Source: CAD feature listing. Evaluate the final solid. Frame: model axes, mm. A direction names the side the tool comes from. Give positions to 0.01 mm unless a question says otherwise; leave off trailing zeros. Order: outer loops, then holes, each group sorted by start corner. A loop starts at its lowest first (then second) coordinate and runs counter-clockwise, first axis right, second up.
from build123d import *

# Parameters (mm, degrees)
PAD_DEPTH       = 4
POCKET_DEPTH    = 1
POCKET001_DEPTH = 3.001


with BuildPart() as part:
    # Sketch → Pad (new body)
    with BuildSketch(Plane.XY):
        with BuildLine():
            Line((0, 0), (50, 0))
            ThreePointArc((50, 0), (62.5, 12.5), (50, 25))
            Line((50, 25), (0, 25))
            ThreePointArc((0, 25), (-12.5, 12.5), (0, 0))
        make_face()
    extrude(amount=PAD_DEPTH)

    # Sketch001 (on Face6 of Pad) → Pocket (cut)
    with BuildSketch(Plane.XY.offset(4)):
        with BuildLine():
            Line((0, 2), (50, 2))
            ThreePointArc((50, 2), (60.5, 12.5), (50, 23))
            Line((50, 23), (0, 23))
            ThreePointArc((0, 23), (-10.5, 12.5), (0, 2))
        make_face()
    extrude(amount=-POCKET_DEPTH, mode=Mode.SUBTRACT)

    # Sketch002 (on Face11 of Pocket) → Pocket001 (cut, through all)
    with BuildSketch(Plane.XY.offset(3)):
        with BuildLine():
            ThreePointArc((-2, 17.5), (-4.5, 20), (-7, 17.5))
            Line((-7, 17.5), (-7, 7.5))
            ThreePointArc((-7, 7.5), (-4.5, 5), (-2, 7.5))
            Line((-2, 7.5), (-2, 17.5))
        make_face()
    extrude(amount=-POCKET001_DEPTH, mode=Mode.SUBTRACT)


solid = part.part
1) Section query A-A on y = 12.5. Output: boundary loops of the cut face in (x, z), and give its area (3 significant figures).
Checks:
outline: (-12.5, 0) - (-7, 0) - (-7, 3) - (-10.5, 3) - (-10.5, 4) - (-12.5, 4) - close; (-2, 0) - (62.5, 0) - (62.5, 4) - (60.5, 4) - (60.5, 3) - (-2, 3) - close
area: 214 mm2
2) Section query C-C on x = -4.5. Output: boundary loops of the cut face in (y, z).
Checks:
outline: (0.84, 0) - (5, 0) - (5, 3) - (3.01, 3) - (3.01, 4) - (0.84, 4) - close; (20, 0) - (24.16, 0) - (24.16, 4) - (21.99, 4) - (21.99, 3) - (20, 3) - close
3) Reachability of faces 1 (the face through (25, 0, 2)), 2 (the face through (25, 13, 3)), 3 (the face through (-4.4, 20, 1.5)) from +Z, -Z, +X, -X, +Y, -Y: full face, straight path, thin tool, end or side. Return the list, or none.
Checks:
face 1: +Z, -Z, +X, -X, -Y
face 2: +Z
face 3: +Z, -Z
4) First-contact query: pin 1 Ø1.5 at (x, y) = (17.5, 13.5) entering from +Z; pin 2 Ø1.5 at (y, z) = (22, 1) entering from -X. Flat tips, straight axial feed; report the tip coordinate or a pass-through.
Checks:
pin 1: stops at z = 3
pin 2: stops at x = -8.93
5) Pull-direction query (X, two-part tool) for faces 4 (the face through (-12.497, 12.775, 1.972)), 5 (the face through (25, 1, 4)), 6 (the face through (-2, 12, 2)); classes: +X half, -X half, draft (parallel to the pull), parting line (faces both ways), or undercut.
Checks:
face 4: -X half
face 5: draft
face 6: undercut
6) Section query B-B on z = 0.95. Output: boundary loops of the cut face in (x, y).
Checks:
outline: (0, 0) - (50, 0) arc R12.5 ccw to (50, 25) - (0, 25) arc R12.5 ccw to start; hole (-7, 7.5) arc R2.5 ccw to (-2, 7.5) - (-2, 17.5) arc R2.5 ccw to (-7, 17.5) - close
7) Ray query, L1, parallel to X at y = 12.5, z = 2.3; L2, parallel to Y at x = 45, z = 3.35; L3, parallel to Z at x = 45.5, y = 9.75. Return the intervals inside material, ascending.
Checks:
L1: x = -12.5 to -7, -2 to 62.5
L2: y = 0 to 2, 23 to 25
L3: z = 0 to 3
8) Section query D-D on x = 6. Output: boundary loops of the cut face in (y, z), and give its area (3 significant figures).
Checks:
outline: (0, 0) - (25, 0) - (25, 4) - (23, 4) - (23, 3) - (2, 3) - (2, 4) - (0, 4) - close
area: 79.0 mm2
